Source: CAD feature listing. Evaluate the final solid. Frame: model axes, mm. Face numbers are marked on the shaded views. A direction names the side the tool comes from. Round coordinates to 2 decimals unless told otherwise and drop trailing zeros. Loops run counter-clockwise (first coordinate to the right, second up) from the corner with the lowest first, then second, coordinate; pieces in that order, holes last. Notation, with made-up numbers: (-29.5, 4) -> (28.5, 4) arc R7 cw to (28.5, 15) -> close; hole circle Ø1 at (48, 6.25). An arc over 180 degrees is marked (long way). Put each result on its own line as item: value. Start each with the question number.
1. Set-up query: the marked faces 1, 2 and 3. Return all of +Z, -Z, +X, -X, +Y, -Y with unobstructed straight access to the full face (end or side cutting, diameter ignored); none if empty.
2. Cut plane D-D (y = 5.08). State how many separate pieces and enclosed holes the cut face has, then the cut area to 3 significant figures.
3. Cut plane C-C (y = 8). Return the cut outline in (x, z), then the cut area to 3 significant figures.
4. Material intervals for L1, parallel to Z at x = 1, y = 1.25; L2, parallel to X at y = 0.5, z = 17; L3, parallel to Y at x = -5.3, z = -15, sorted ascending.
5. Draft query along Z for the marked faces 4, 5 and 6. Return one class per face: pulls with the +Z half, pulls with the -Z half, needs draft (parallel to the pull), parting line crosses it, or undercut.
6. Cut plane B-B (z = 15). Return the cut outline in (x, y), then the cut area to 3 significant figures.
7. Contact query for flat-ended pins moving along their axis: pin 1 (3 mm diameter, centred on y = 7, z = 13.5, fed in from -X); pin 2 (5 mm diameter, centred on y = 6.5, z = 17, fed in from +X); pin 3 (5 mm diameter, centred on y = 7, z = 5.5, fed in from -X). Output: stop coordinate, or through.
8. Cut plane A-A (y = 1.75). Return the cut outline in (x, z), then the cut area to 3 significant figures.
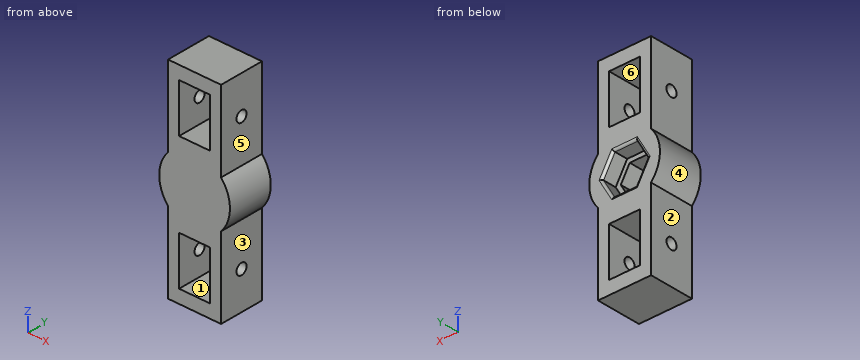
Autodesk Inventor part; units mm, degrees
ref_plane "YZ Plane" through (0, 0, 0) normal (1, 0, 0) x (0, 1, 0)
ref_plane "XZ Plane" through (0, 0, 0) normal (0, 1, 0) x (-1, 0, 0)
ref_plane "XY Plane" through (0, 0, 0) normal (0, 0, 1) x (1, 0, 0)
sketch "스케치1" plane through (0, 0, 0) normal (0, 1, 0) x (-1, 0, 0)
  circle A0 centre (0, 0) radius 8
  dimension "d0" = 16
extrude "돌출1" add sketch "스케치1" along normal blind 10.16
sketch "스케치2" plane through (0, 10.16, 0) normal (0, 1, 0) x (1, 0, 0)
  circle A0 centre (0, 0) radius 4.5
  line L0 (2.5981, -4.5) -> (-2.5981, -4.5)
  line L1 (-2.5981, -4.5) -> (-5.1962, 0)
  line L2 (-5.1962, 0) -> (-2.5981, 4.5)
  line L3 (-2.5981, 4.5) -> (2.5981, 4.5)
  line L4 (2.5981, 4.5) -> (5.1962, 0)
  line L5 (5.1962, 0) -> (2.5981, -4.5)
  dimension "d3" = 9
sketch "스케치3" plane through (0, 0, 0) normal (0, -1, 0) x (1, 0, 0)
  line L0 (-3, 9.5) -> (3, 9.5)
  line L1 (3, 9.5) -> (3, 20.5)
  line L2 (3, 20.5) -> (-3, 20.5)
  line L3 (-3, 20.5) -> (-3, 9.5)
  line L4 (-3, 9.5) -> (3, 20.5) construction
  line L5 (3, 9.5) -> (-3, 20.5) construction
  line L6 (0, 0) -> (5.3002, 0)
  line L7 (-3, -9.5) -> (3, -9.5)
  line L8 (3, -9.5) -> (3, -20.5)
  line L9 (3, -20.5) -> (-3, -20.5)
  line L10 (-3, -20.5) -> (-3, -9.5)
  line L11 (-3, -9.5) -> (3, -20.5) construction
  line L12 (3, -9.5) -> (-3, -20.5) construction
  line L13 (6, 23.5) -> (-6, 23.5)
  line L14 (-6, 23.5) -> (-6, -23.5)
  line L15 (-6, -23.5) -> (6, -23.5)
  line L16 (6, -23.5) -> (6, 23.5)
  line L17 (6, 23.5) -> (-6, -23.5) construction
  line L18 (-6, 23.5) -> (6, -23.5) construction
  circle A0 centre (0, 0) radius 8
  point P0 (0, 15)
  point P1 (0, -15)
  point P2 (6, 5.2915)
  point P3 (-6, 5.2915)
  point P4 (-6, -5.2915)
  point P5 (6, -5.2915)
  dimension "d7" = 6
  dimension "d8" = 11
  dimension "d10" = 15
  dimension "d11" = 3
  dimension "d12" = 3
extrude "돌출3" add sketch "스케치3" against normal blind 10.16 contours L3 L2 L1 L0 | L7 L8 L9 L10 | L16 A0 L14 L13 | L16 L15 L14 A0
extrude "돌출4" cut sketch "스케치2" against normal blind 8
sketch "스케치4" plane through (0, 2.16, 0) normal (0, 1, 0) x (1, 0, 0)
  line L0 (2.0207, 3.5) -> (4.0415, 0)
  line L1 (4.0415, 0) -> (2.0207, -3.5)
  line L2 (2.0207, -3.5) -> (-2.0207, -3.5)
  line L3 (-2.0207, -3.5) -> (-4.0415, 0)
  line L4 (-4.0415, 0) -> (-2.0207, 3.5)
  line L5 (-2.0207, 3.5) -> (2.0207, 3.5)
  line L6 (-2.5981, 4.5) -> (2.5981, 4.5)
  line L7 (2.5981, 4.5) -> (5.1962, 0)
  line L8 (-2.5981, 4.5) -> (2.5981, 4.5)
  line L9 (-5.1962, 0) -> (-2.5981, 4.5)
  line L10 (-2.5981, -4.5) -> (-5.1962, 0)
  line L11 (2.5981, -4.5) -> (-2.5981, -4.5)
  line L12 (5.1962, 0) -> (2.5981, -4.5)
  point P0 (0, 0)
  point P1 (0, 0)
  dimension "d17" = 1
extrude "돌출5" add sketch "스케치4" along normal blind 4.5
fillet "모깎기2" radius 0.5 6 edges at (3.8971, 10.16, -2.25) (3.8971, 10.16, 2.25) (0, 10.16, -4.5) (0, 10.16, 4.5) (-3.8971, 10.16, 2.25) (-3.8971, 10.16, -2.25)
sketch "스케치6" plane through (0, 10.16, 0) normal (0, 1, 0) x (1, 0, 0)
  line L0 (-3.5, -9.5) -> (3.5, -9.5)
  line L1 (3.5, -9.5) -> (3.5, -20.5)
  line L2 (3.5, -20.5) -> (-3.5, -20.5)
  line L3 (-3.5, -20.5) -> (-3.5, -9.5)
  line L4 (-3.5, -9.5) -> (3.5, -20.5) construction
  line L5 (3.5, -9.5) -> (-3.5, -20.5) construction
  line L6 (-6, -23.5) -> (6, -23.5)
  line L7 (6, -23.5) -> (6, -5.2915)
  line L8 (2.8868, -5) -> (5.7735, 0)
  line L9 (-5.1962, 0) -> (-5.7735, 0)
  line L10 (5.7735, 0) -> (-5.7735, 0)
  line L11 (-3.5, 9.5) -> (3.5, 9.5)
  line L12 (3.5, 9.5) -> (3.5, 20.5)
  line L13 (3.5, 20.5) -> (-3.5, 20.5)
  line L14 (-3.5, 20.5) -> (-3.5, 9.5)
  line L15 (-3.5, 9.5) -> (3.5, 20.5) construction
  line L16 (3.5, 9.5) -> (-3.5, 20.5) construction
  line L17 (-6, 23.5) -> (6, 23.5)
  line L18 (6, 23.5) -> (6, 5.2915)
  point P0 (0, 0)
  point P1 (0, -15)
  point P2 (0, 15)
  point P3 (0, 0)
  dimension "d21" = 7
  dimension "d22" = 11
  dimension "d23" = 3
extrude "돌출6" cut sketch "스케치6" against normal blind 10.16
sketch "스케치7" plane through (-6, 0, 5.2915) normal (-1, 0, 0) x (0, 0, 1)
  line L0 (4.2085, 10.16) -> (15.2085, 10.16)
  line L1 (4.2085, 10.16) -> (4.2085, 0)
  line L2 (15.2085, 0) -> (4.2085, 0)
  line L3 (15.2085, 10.16) -> (15.2085, 0)
  line L4 (-25.7915, 10.16) -> (-14.7915, 10.16)
  line L5 (-25.7915, 10.16) -> (-25.7915, 0)
  line L6 (-14.7915, 0) -> (-25.7915, 0)
  line L7 (-14.7915, 10.16) -> (-14.7915, 0)
  circle A0 centre (9.7085, 5.08) radius 1.25
  line L8 (-10.2915, 10.16) -> (-5.2915, 10.16)
  line L9 (-5.2915, 0) -> (-5.2915, 10.16)
  circle A1 centre (-20.2915, 5.08) radius 1.25
  point P0 (15.2085, 5.08)
  point P1 (9.7085, 0)
  dimension "d27" = 2.5
extrude "돌출7" cut sketch "스케치7" against normal up to surface (12 mm away) contours A0 | A1
properties part number "Tensile_test_top_adapter"
Solution:
1. face 1: +Y, -Y
1. face 2: -Z, -X, +Y, -Y
1. face 3: -Z, +X, +Y, -Y
2. separate pieces: 3
2. enclosed holes: 1
2. area: 372 mm^2
3. outline: (-6, -23.5) -> (6, -23.5) -> (6, -5.29) arc R8 ccw to (6, 5.29) -> (6, 23.5) -> (-6, 23.5) -> (-6, 5.29) arc R8 ccw to (-6, -5.29) -> close; hole (-5.2, 0) -> (-2.6, -4.5) -> (2.6, -4.5) -> (5.2, 0) -> (2.6, 4.5) -> (-2.6, 4.5) -> close; hole (-3.5, -20.5) -> (3.5, -20.5) -> (3.5, -9.5) -> (-3.5, -9.5) -> close; hole (-3.5, 9.5) -> (3.5, 9.5) -> (3.5, 20.5) -> (-3.5, 20.5) -> close
3. area: 369 mm^2
4. L1: z = -23.5 to -20.5, -9.5 to 9.5, 20.5 to 23.5
4. L2: x = -6 to -3.5, 3.5 to 6
4. L3: y = 0 to 3.83, 6.33 to 10.16
5. face 4: parting line crosses it
5. face 5: needs draft
5. face 6: undercut
6. outline: (-6, 0) -> (-3.5, 0) -> (-3.5, 3.83) -> (-6, 3.83) -> close; (-6, 6.33) -> (-3.5, 6.33) -> (-3.5, 10.16) -> (-6, 10.16) -> close; (3.5, 0) -> (6, 0) -> (6, 3.83) -> (3.5, 3.83) -> close; (3.5, 6.33) -> (6, 6.33) -> (6, 10.16) -> (3.5, 10.16) -> close
6. area: 38.3 mm^2
7. pin 1: stops at x = -6
7. pin 2: stops at x = 6
7. pin 3: stops at x = -7.42
8. outline: (-6, -23.5) -> (6, -23.5) -> (6, -5.29) arc R8 ccw to (6, 5.29) -> (6, 23.5) -> (-6, 23.5) -> (-6, 5.29) arc R8 ccw to (-6, -5.29) -> close; hole (-3.5, -20.5) -> (3.5, -20.5) -> (3.5, -9.5) -> (-3.5, -9.5) -> close; hole (-3.5, 9.5) -> (3.5, 9.5) -> (3.5, 20.5) -> (-3.5, 20.5) -> close
8. area: 439 mm^2
